The listing builds one solid part. Answer for the finished solid, in the listing's coordinates (mm). Face numbers are marked on the shaded views. A direction names the side the tool comes from. Give positions to 0.01 mm unless a question says otherwise; leave off trailing zeros. Write each loop counter-clockwise with the first axis right and the second up, starting at its lowest first coordinate (ties: lowest second). Pieces come first, ordered by that corner, then holes. Notation, with made-up numbers: (31.25, -9.5) -> (47.25, -9.5) arc R33 ccw to (47.25, 19.5) -> close; hole circle Ø9 at (10, -10). An arc over 180 degrees is marked (long way). Write each question's results on one line, items separated by ' | '. Start each with the question number.
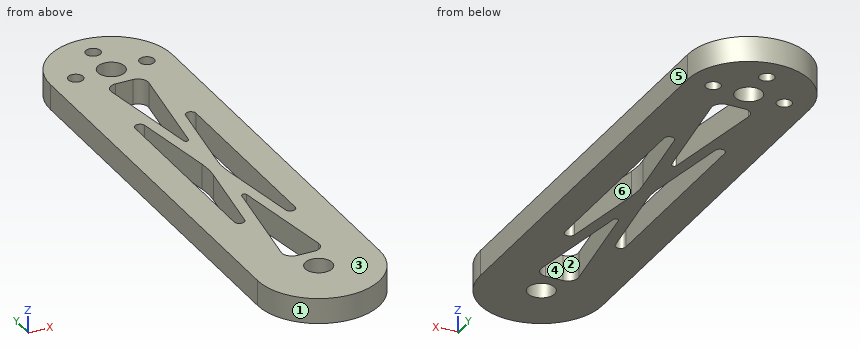
from build123d import *

# Parameters (mm, degrees)
SKETCH_1_R      = 2.65
SKETCH_1_R_2    = 1.45
EXTRUDE_1_DEPTH = 5


with BuildPart() as part:
    # 草图1 → 凸台-拉伸1 (new body)
    with BuildSketch(Plane.XY):
        with BuildLine():
            Line((-12, 40), (-12, -40))
            ThreePointArc((-12, -40), (0, -52), (12, -40))
            Line((12, -40), (12, 40))
            ThreePointArc((12, 40), (0, 52), (-12, 40))
        make_face()
        with Locations((0, 40)):
            Circle(SKETCH_1_R, mode=Mode.SUBTRACT)
        with Locations((0, -40)):
            Circle(SKETCH_1_R, mode=Mode.SUBTRACT)
        with Locations((7, 40)):
            Circle(SKETCH_1_R_2, mode=Mode.SUBTRACT)
        with Locations((-7, 40)):
            Circle(SKETCH_1_R_2, mode=Mode.SUBTRACT)
        with Locations((0, 47)):
            Circle(SKETCH_1_R_2, mode=Mode.SUBTRACT)
        with BuildLine():
            Line((-1.684371732, 35), (1.684371732, 35))
            ThreePointArc((1.684371732, 35), (3.19797273, 34.307291865), (3.663090003, 32.709012019))
            Line((3.663090003, 32.709012019), (0.494679568, 11.16382106))
            ThreePointArc((0.494679568, 11.16382106), (0, 10.736568055), (-0.494679568, 11.16382106))
            Line((-0.494679568, 11.16382106), (-3.663090003, 32.709012019))
            ThreePointArc((-3.663090003, 32.709012019), (-3.19797273, 34.307291865), (-1.684371732, 35))
        make_face(mode=Mode.SUBTRACT)
        with BuildLine():
            Line((6, 19.095781345), (6, -19.163256412))
            ThreePointArc((6, -19.163256412), (5.073630361, -20.160542013), (4.01084286, -19.31011741))
            Line((4.01084286, -19.31011741), (1.482419396, -2.280353461))
            ThreePointArc((1.482419396, -2.280353461), (1.319777526, -0.083000608), (1.480789762, 2.114472259))
            Line((1.480789762, 2.114472259), (4.010734218, 19.241908728))
            ThreePointArc((4.010734218, 19.241908728), (5.073260555, 20.09309418), (6, 19.095781345))
        make_face(mode=Mode.SUBTRACT)
        with BuildLine():
            Line((-1.684371732, -35), (1.684371732, -35))
            ThreePointArc((1.684371732, -35), (3.19839114, -34.306807267), (3.662903296, -32.707745233))
            Line((3.662903296, -32.707745233), (0.494632891, -11.258914622))
            ThreePointArc((0.494632891, -11.258914622), (0, -10.831978314), (-0.494632891, -11.258914622))
            Line((-0.494632891, -11.258914622), (-3.662903296, -32.707745233))
            ThreePointArc((-3.662903296, -32.707745233), (-3.19839114, -34.306807267), (-1.684371732, -35))
        make_face(mode=Mode.SUBTRACT)
        with BuildLine():
            Line((-6, -19.163256412), (-6, 19.095781345))
            ThreePointArc((-6, 19.095781345), (-5.073260555, 20.09309418), (-4.010734218, 19.241908728))
            Line((-4.010734218, 19.241908728), (-1.480789762, 2.114472259))
            ThreePointArc((-1.480789762, 2.114472259), (-1.319777526, -0.083000608), (-1.482419396, -2.280353461))
            Line((-1.482419396, -2.280353461), (-4.01084286, -19.31011741))
            ThreePointArc((-4.01084286, -19.31011741), (-5.073630361, -20.160542013), (-6, -19.163256412))
        make_face(mode=Mode.SUBTRACT)
    extrude(amount=EXTRUDE_1_DEPTH)


solid = part.part
1. Each of these flat-tipped pins is pushed along its axis until it touches: pin 1 Ø1.7 at (x, y) = (7, 40) entering from +Z; pin 2 Ø6 at (x, y) = (0, -40) entering from -Z. Where does it stop, or does it pass through?
2. Section A-A (z = 3.65) is taken. Give the number of separate pieces and of enclosed holes in the cut face, then the cut area to 3 significant figures.
3. A tool of negligible diameter and unlimited length cuts with its end or side. For the marked faces 5 and 6, from which of +Z, -Z, +X, -X, +Y, -Y can it reach the whole face along a straight path? Write none if from no direction.
4. Section D-D (y = -7.5) is taken. Write down the section's boundary in (x, z).
5. Section C-C (y = 29.5) is taken. Write down the section's boundary in (x, z), then the cut area to 3 significant figures.
6. Section B-B (x = 7) is taken. Write down the section's boundary in (y, z), then the cut area to 3 significant figures.
7. The mould has two halves that part along Y. Classify the marked faces 1, 2, 3 and 4: pulls with the +Y half, pulls with the -Y half, needs draft (parallel to the pull), parting line crosses it, or undercut.
8. Consider probe 1 along Y at (x, z) = (0, 3.9); probe 2 along Y at (x, z) = (7, 1.9); probe 3 along X at (y, z) = (1, 1.45). Determine where each line is inside the solid, lowest interval first. Write a range as [from, to].
Results:
1) pin 1: passes through | pin 2: stops at z = 0
2) separate pieces: 1 | enclosed holes: 9 | area: 1,830 mm²
3) face 5: +Z, -Z, +X, +Y, -Y | face 6: +Z, -Z
4) outline: (-12, 0) -> (-6, 0) -> (-6, 5) -> (-12, 5) -> close; (-2.26, 0) -> (2.26, 0) -> (2.26, 5) -> (-2.26, 5) -> close; (6, 0) -> (12, 0) -> (12, 5) -> (6, 5) -> close
5) outline: (-12, 0) -> (-3.19, 0) -> (-3.19, 5) -> (-12, 5) -> close; (3.19, 0) -> (12, 0) -> (12, 5) -> (3.19, 5) -> close | area: 88.1 mm²
6) outline: (-49.75, 0) -> (38.55, 0) -> (38.55, 5) -> (-49.75, 5) -> close; (41.45, 0) -> (49.75, 0) -> (49.75, 5) -> (41.45, 5) -> close | area: 483 mm²
7) face 1: pulls with the -Y half | face 2: undercut | face 3: needs draft | face 4: undercut
8) probe 1: y = [-52, -42.65], [-37.35, -35], [-10.83, 10.74], [35, 37.35], [42.65, 45.55], [48.45, 52] | probe 2: y = [-49.75, 38.55], [41.45, 49.75] | probe 3: x = [-12, -6], [-1.36, 1.36], [6, 12]
